Verification items for this drawing (mm, ordinates from the low corner). A direction names the side the tool comes from. Coordinates: 2 decimals unless noted, no trailing zeros. Answer as a JSON object with one key per item and string values. Group by question number.
(1) Access from +Z, -Z, +X, -X, +Y, -Y to the whole of each face (thin tool, end or side, straight path). Record for the marked faces 4 and 5.
(2) Mould release check, pull along Z, two halves, no side actions. Record for the marked faces 1, 2 and 3: released by +Z, released by -Z, zero draft, split by the parting line, or undercut.
(3) Gauge pin test, flat ends, axial feed: pin 1 Ø2 at (x, z) = (32, 10) entering from -Y; pin 2 Ø1.5 at (y, z) = (3, 21.5) entering from +X (1 decimal). Record the tip position at first contact, or that the pin passes through.
(4) Material ranges on line 1 (X direction, y = 7.75, z = 25.4) (1 decimal); line 2 (X direction, y = 12.75, z = 25.5); line 3 (Z direction, x = 23, y = 20), recorded low to high.
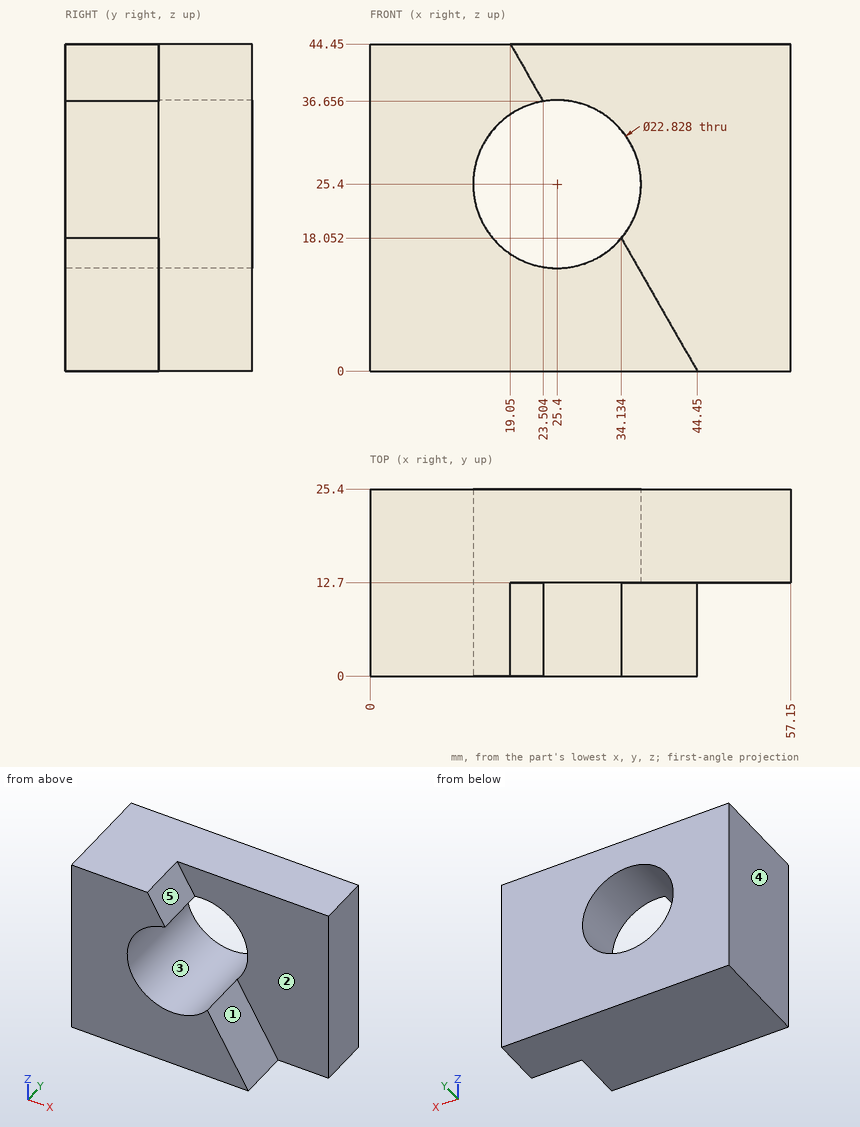
Taken from the geometry:
{
 "1": {"face 4": "+Z, -Z, -X, +Y, -Y", "face 5": "+Z, +X, -Y"},
 "2": {"face 1": "released by +Z", "face 2": "zero draft", "face 3": "undercut"},
 "3": {"pin 1": "stops at y = 0", "pin 2": "stops at x = 15"},
 "4": {"line 1": "x = 0 to 14", "line 2": "x = 0 to 13.99, 36.81 to 57.15", "line 3": "z = 0 to 14.24, 36.56 to 44.45"}
}
